Can you work these out from the model? Positions are in its coordinate system, mm. Round coordinates to 2 decimals unless told otherwise and drop trailing zeros. Order: outer loops, then holes, each group sorted by start corner. A loop starts at its lowest first (then second) coordinate and runs counter-clockwise, first axis right, second up.
Q1. If we section it at D-D (x = -12): Please give me the cut outline in (y, z), plus the area to 3 significant figures.
Q2. If we section it at C-C (y = -29): Please give me the cut outline in (x, z), plus the area to 3 significant figures.
Q3. If we section it at A-A (y = 0): Please give me the cut outline in (x, z).
Q4. Will this pin go through, and if not, where does the flat tip stop? P1, Ø2, axis at x = 0, z = 12, coming from the +Y side.
Q5. If I drill on line 1 (Y direction, x = 0, z = 11); line 2 (X direction, y = -19.5, z = 17); line 3 (Y direction, x = -1, z = 19.5), over which ranges is the centre line in solid material (lowest first)?
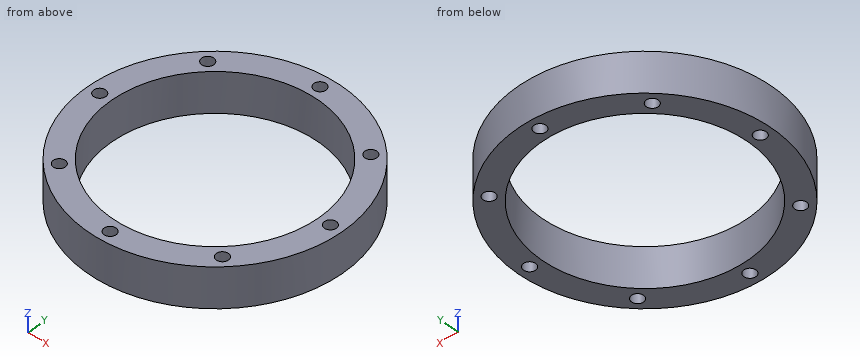
from build123d import *

# Parameters (mm, degrees)
CYLINDER188_R               = 1.5
CYLINDER188_DEPTH           = 30
CYLINDER188_PLACEMENT_ANGLE = 45
CYLINDER189_R               = 1.5
CYLINDER189_DEPTH           = 30
CYLINDER190_R               = 1.5
CYLINDER190_DEPTH           = 30
CYLINDER190_PLACEMENT_ANGLE = 135
CYLINDER191_R               = 1.5
CYLINDER191_DEPTH           = 30
CYLINDER192_R               = 1.5
CYLINDER192_DEPTH           = 30
CYLINDER192_PLACEMENT_ANGLE = 225
CYLINDER193_R               = 1.5
CYLINDER193_DEPTH           = 30
CYLINDER194_R               = 1.5
CYLINDER194_DEPTH           = 30
CYLINDER194_PLACEMENT_ANGLE = 45
CYLINDER187_R               = 1.5
CYLINDER187_DEPTH           = 30
TUBE012_R                   = 32
TUBE012_R_2                 = 26
TUBE012_DEPTH               = 10


with BuildPart() as obj1:
    # Cylinder188 → Cylinder188 (new body)
    with BuildSketch(Plane.XY):
        Circle(CYLINDER188_R)
    extrude(amount=CYLINDER188_DEPTH)


with BuildPart() as obj1_1:
    # Cylinder188 placement: moved
    add(obj1.part.moved(Location((20.506097, -20.506097, 0))).rotate(Axis((20.506097, -20.506097, 0), (0, 0, 1)), CYLINDER188_PLACEMENT_ANGLE))


with BuildPart() as obj2:
    # Cylinder189 → Cylinder189 (new body)
    with BuildSketch(Plane(origin=(29, 0, 0), x_dir=(0, 1, 0), z_dir=(0, 0, 1))):
        Circle(CYLINDER189_R)
    extrude(amount=CYLINDER189_DEPTH)


with BuildPart() as obj3:
    # Cylinder190 → Cylinder190 (new body)
    with BuildSketch(Plane.XY):
        Circle(CYLINDER190_R)
    extrude(amount=CYLINDER190_DEPTH)


with BuildPart() as obj3_1:
    # Cylinder190 placement: moved
    add(obj3.part.moved(Location((20.506097, 20.506097, 0))).rotate(Axis((20.506097, 20.506097, 0), (0, 0, 1)), CYLINDER190_PLACEMENT_ANGLE))


with BuildPart() as obj4:
    # Cylinder191 → Cylinder191 (new body)
    with BuildSketch(Plane(origin=(0, 29, 0), x_dir=(-1, 0, 0), z_dir=(0, 0, 1))):
        Circle(CYLINDER191_R)
    extrude(amount=CYLINDER191_DEPTH)


with BuildPart() as obj5:
    # Cylinder192 → Cylinder192 (new body)
    with BuildSketch(Plane.XY):
        Circle(CYLINDER192_R)
    extrude(amount=CYLINDER192_DEPTH)


with BuildPart() as obj5_1:
    # Cylinder192 placement: moved
    add(obj5.part.moved(Location((-20.506097, 20.506097, 0))).rotate(Axis((-20.506097, 20.506097, 0), (0, 0, 1)), CYLINDER192_PLACEMENT_ANGLE))


with BuildPart() as obj6:
    # Cylinder193 → Cylinder193 (new body)
    with BuildSketch(Plane(origin=(-29, 0, 0), x_dir=(0, -1, 0), z_dir=(0, 0, 1))):
        Circle(CYLINDER193_R)
    extrude(amount=CYLINDER193_DEPTH)


with BuildPart() as obj7:
    # Cylinder194 → Cylinder194 (new body)
    with BuildSketch(Plane.XY):
        Circle(CYLINDER194_R)
    extrude(amount=CYLINDER194_DEPTH)


with BuildPart() as obj7_1:
    # Cylinder194 placement: moved
    add(obj7.part.moved(Location((-20.506097, -20.506097, 0))).rotate(Axis((-20.506097, -20.506097, 0), (0, 0, -1)), CYLINDER194_PLACEMENT_ANGLE))


with BuildPart() as compound544:
    # Cylinder187 → Cylinder187 (new body)
    with BuildSketch(Plane(origin=(0, -29, 0), x_dir=(1, 0, 0), z_dir=(0, 0, 1))):
        Circle(CYLINDER187_R)
    extrude(amount=CYLINDER187_DEPTH)

    # Compound544: union obj1, obj2, obj3, obj4, obj5, obj6, obj7
    add(obj1_1.part)
    add(obj2.part)
    add(obj3_1.part)
    add(obj4.part)
    add(obj5_1.part)
    add(obj6.part)
    add(obj7_1.part)


with BuildPart() as cut318:
    # Tube012 → Tube012 (new body)
    with BuildSketch(Plane.XY.offset(10)):
        Circle(TUBE012_R)
        Circle(TUBE012_R_2, mode=Mode.SUBTRACT)
    extrude(amount=TUBE012_DEPTH)

    # Cut318: cut Compound544
    add(compound544.part, mode=Mode.SUBTRACT)


solid = cut318.part
Solution:
1. outline: (-29.66, 10) - (-23.07, 10) - (-23.07, 20) - (-29.66, 20) - close; (23.07, 10) - (29.66, 10) - (29.66, 20) - (23.07, 20) - close
1. area: 132 mm2
2. outline: (-13.53, 10) - (-1.5, 10) - (-1.5, 20) - (-13.53, 20) - close; (1.5, 10) - (13.53, 10) - (13.53, 20) - (1.5, 20) - close
2. area: 241 mm2
3. outline: (-32, 10) - (-30.5, 10) - (-30.5, 20) - (-32, 20) - close; (-27.5, 10) - (-26, 10) - (-26, 20) - (-27.5, 20) - close; (26, 10) - (27.5, 10) - (27.5, 20) - (26, 20) - close; (30.5, 10) - (32, 10) - (32, 20) - (30.5, 20) - close
4. P1: stops at y = 32
5. line 1: y = -32 to -30.5, -27.5 to -26, 26 to 27.5, 30.5 to 32
5. line 2: x = -25.37 to -21.62, -19.39 to -17.2, 17.2 to 19.39, 21.62 to 25.37
5. line 3: y = -31.98 to -30.12, -27.88 to -25.98, 25.98 to 27.88, 30.12 to 31.98
